The model under review builds one solid part; all positions refer to its coordinate system, in mm. Face numbers are marked on the shaded views. Round coordinates to 2 decimals unless told otherwise and drop trailing zeros. Order: outer loops, then holes, each group sorted by start corner. A loop starts at its lowest first (then second) coordinate and runs counter-clockwise, first axis right, second up. Notation, with made-up numbers: (-26, 85.5) -> (0, 85.5) arc R25 ccw to (0, 118.5) -> close; hole circle Ø5 at (6.5, 64.5). An arc over 180 degrees is marked (long way). Use a Markdown table: item, result. Add a question column.
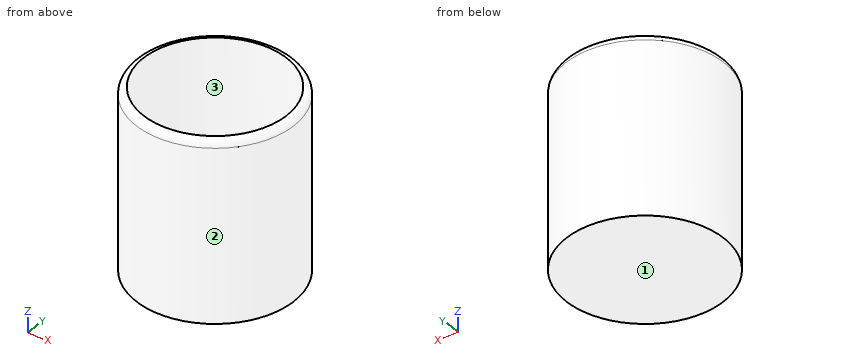
```python
from build123d import *

# Parameters (mm, degrees)
F0_R     = 11
F1_DEPTH = 25
F2_R     = 10
F3_DEPTH = 22
F4_SIZE  = 0.5
F5_R     = 0.99999


# Not quite as in the source:
# - a fillet or chamfer is up to 0.001 mm smaller than in the source, because OpenCascade refuses the exact size


with BuildPart() as f1:
    # F0 (on Top) → F1 (new body)
    with BuildSketch(Plane.XY):
        Circle(F0_R)
    extrude(amount=F1_DEPTH)

    # F2 (on face) → F3 (cut)
    with BuildSketch(Plane.XY.offset(25)):
        Circle(F2_R)
    extrude(amount=-F3_DEPTH, mode=Mode.SUBTRACT)

    # F4
    f4_edges = [f1.edges().sort_by_distance(p)[0] for p in [
        (-10, 0, 3),
    ]]
    chamfer(f4_edges, length=F4_SIZE)

    # F5 (radius 1 in the source; OpenCascade refuses exactly that, so slightly less here)
    f5_edges = [f1.edges().sort_by_distance(p)[0] for p in [
        (-11, 0, 25),
    ]]
    fillet(f5_edges, radius=F5_R)


solid = f1.part
```
Q1. Add section B-B (z = 6). Write out the cut boundary in (x, y), then the cut area to 3 significant figures.
Q2. Insertion check: pin 1 (3 mm diameter, centred on x = -4.5, z = 19, fed in from +Y); pin 2 (1 mm diameter, centred on y = -4.5, z = 14, fed in from -X); pin 3 (5 mm diameter, centred on x = -5.5, z = 6, fed in from -Y). Each pin has a flat end and moves straight along its axis. Give the tip position at first contact, or say it passes through.
Q3. Mouldability with a two-part tool opening along Y and no side actions: class the marked faces 1, 2 and 3 as pulls with the +Y half, pulls with the -Y half, needs draft (parallel to the pull), parting line crosses it, or undercut.
Q4. Wall thickness on line 1 (Y direction, x = 0, z = 15.5); line 2 (Z direction, x = -1.25, y = -7.5); line 3 (Z direction, x = 8.5, y = 5.5): over which ranges is each line inside the solid? List them lowest first. Write a range as [from, to].
Report:
| question | item | result |
|---|---|---|
| 1 | outline | circle Ø22 at (0, 0); hole circle Ø20 at (0, 0) |
| 1 | area | 66.0 mm² |
| 2 | pin 1 | stops at y = 10.58 |
| 2 | pin 2 | stops at x = -10.25 |
| 2 | pin 3 | stops at y = -10.58 |
| 3 | face 1 | needs draft |
| 3 | face 2 | parting line crosses it |
| 3 | face 3 | undercut |
| 4 | line 1 | y = [-11, -10], [10, 11] |
| 4 | line 2 | z = [0, 3] |
| 4 | line 3 | z = [0, 24.99] |
